Design review of the part built by this model. Coordinates are the model's own, in mm. A direction names the side the tool comes from. Give positions to 0.01 mm unless a question says otherwise; leave off trailing zeros. Write each loop counter-clockwise with the first axis right and the second up, starting at its lowest first coordinate (ties: lowest second). Pieces come first, ordered by that corner, then holes. Notation, with made-up numbers: M -38,66 L -29,66 A7 cw -29,78 Z; hole C -3,76.25 d3. An arc over 180 degrees is marked long. Answer in a Markdown table with one row per item.
```python
from build123d import *

# Parameters (mm, degrees)
F1_DEPTH = 63.5
F0_W     = 25.4
F0_H     = 19.05
F2_DEPTH = 25.4
F3_DEPTH = 7.9375
F5_R     = 6.35
F6_R     = 12.7
F7_DEPTH = 76.201
F8_R     = 2.54
F9_SIZE  = 2.54


with BuildPart() as f1:
    # F0 (on Front) → F1 (new body, symmetric)
    with BuildSketch(Plane.XZ):
        Polygon((-41.275, -9.525), (41.275, -9.525), (41.275, 9.525), (22.225, 9.525), (-41.275, 9.525), align=None)
    extrude(amount=F1_DEPTH, both=True)

    # F0 (on Front) → F2 (join, symmetric)
    with BuildSketch(Plane.XZ):
        with BuildLine():
            Line((22.225, 9.525), (41.275, 9.525))
            Line((41.275, 9.525), (41.275, 27.0002))
            ThreePointArc((41.275, 27.0002), (45.9246798487, 38.2255201513), (57.15, 42.8752))
            Line((57.15, 42.8752), (60.325, 42.8752))
            Line((60.325, 42.8752), (60.325, 61.9252))
            Line((60.325, 61.9252), (57.15, 61.9252))
            add(Edge.make_bspline(
                [(57.15, 61.9252), (56.6797844251, 61.9165132353), (56.2111060081, 61.9070782377), (55.7439674805, 61.896886054)],
                knots=[0, 0, 0, 0, 0.9174307887, 0.9174307887, 0.9174307887, 0.9174307887], degree=3))
            ThreePointArc((55.7439674805, 61.896886054), (31.9620930728, 51.1936902325), (22.225, 27.0002))
            Line((22.225, 27.0002), (22.225, 9.525))
        make_face()
        with Locations((73.025, 52.4002)):
            Rectangle(F0_W, F0_H)
    extrude(amount=F2_DEPTH, both=True)

    # F0 (on Front) → F3 (join, symmetric)
    with BuildSketch(Plane.XZ):
        with BuildLine():
            add(Edge.make_bspline(
                [(55.7439674805, 61.896886054), (-0.5649096696, 60.6683202624), (-34.4993601081, 48.437924622), (-41.275, 9.525)],
                knots=[0.9174307887, 0.9174307887, 0.9174307887, 0.9174307887, 111.5045361635, 111.5045361635, 111.5045361635, 111.5045361635], degree=3))
            Line((-41.275, 9.525), (22.225, 9.525))
            Line((22.225, 9.525), (22.225, 27.0002))
            ThreePointArc((22.225, 27.0002), (31.9620930728, 51.1936902325), (55.7439674805, 61.896886054))
        make_face()
    extrude(amount=F3_DEPTH, both=True)

    # F0 (on Front) → F4 (revolve)
    with BuildSketch(Plane.XZ):
        Polygon((85.725, 61.9252), (85.725, 42.8752), (85.725, 38.1), (111.125, 38.1), (111.125, 66.675), (85.725, 66.675), align=None)
    revolve(axis=Axis((85.725, 0, 52.3875), (0, 0, 1)))

    # F5
    f5_edges = [f1.edges().sort_by_distance(p)[0] for p in [
        (-41.275, -63.5, 0),
        (41.275, -63.5, 0),
        (41.275, 63.5, 0),
        (-41.275, 63.5, 0),
    ]]
    fillet(f5_edges, radius=F5_R)

    # F6 (on face) → F7 (cut, through all)
    with BuildSketch(Plane.XY.offset(66.675)):
        with Locations((85.725, 0)):
            Circle(F6_R)
    extrude(amount=-F7_DEPTH, mode=Mode.SUBTRACT)

    # F8
    f8_edges = [f1.edges().sort_by_distance(p)[0] for p in [
        (60.325, 0, 66.675),
        (60.325, 0, 38.1),
    ]]
    fillet(f8_edges, radius=F8_R)

    # F9
    f9_edges = [f1.edges().sort_by_distance(p)[0] for p in [
        (73.025, 0, 66.675),
        (73.025, 0, 38.1),
    ]]
    chamfer(f9_edges, length=F9_SIZE)


solid = f1.part
```
1) The part is to be moulded in two halves that separate along Y. For faces 1 (the face through (91.642, -11.376, 40.517)), 2 (the face through (46, 25.4, 42)), 3 (the face through (1, -36, 9.525)), say which applies: released by +Y, released by -Y, zero draft, split by the parting line, or undercut.
Geometry says:
| item | result |
|---|---|
| face 1 | undercut |
| face 2 | released by +Y |
| face 3 | zero draft |
2) For faces 4 (the face through (81, -15, 38.1)), 5 (the face through (46, -25.4, 42)), 6 (the face through (32.22, -16.79, 51.46)), 7 (the face through (45.8, -0.4, 38.1)), 8 (the face through (60, 2, 42.875)), list the 3-axis set-ups (+Z, -Z, +X, -X, +Y, -Y) from which the entire face can be reached by the end or side of a thin tool; tool diameter is ignored.
Geometry says:
| item | result |
|---|---|
| face 4 | -Z, +X, +Y, -Y |
| face 5 | +Z, +X, -X, -Y |
| face 6 | +Z, -X, -Y |
| face 7 | -Z, +Y, -Y |
| face 8 | -Z |
3) Insertion check: P1, Ø14.5, axis at x = 65, y = 8.5, coming from the -Z side; P2, Ø12, axis at x = 77.5, z = 50.5, coming from the +Y side; P3, Ø2, axis at x = -22, z = 27.5, coming from the -Y side. Each pin has a flat end and moves straight along its axis. Give the tip position at first contact, or say it passes through.
Geometry says:
| item | result |
|---|---|
| P1 | z = 38.1 |
| P2 | y = 25.4 |
| P3 | y = -7.94 |
4) Add section A-A (y = -36). Write out the cut boundary in (x, z) (3 decimals), and give its area (3 significant figures).
Geometry says:
| item | result |
|---|---|
| outline | M -41.275,-9.525 L 41.275,-9.525 L 41.275,9.525 L -41.275,9.525 Z |
| area | 1,570 mm^2 |
5) To check wall thickness, follow probe 1 along X at (y, z) = (21, 14.5) (3 decimals); probe 2 along Z at (x, y) = (35, -46.5) (3 decimals); probe 3 along Y at (x, z) = (25.5, 59.5). State the ranges of each line that lie inside material, in increasing order. Write a range as [from, to].
Geometry says:
| item | result |
|---|---|
| probe 1 | [22.225, 41.275] |
| probe 2 | [-9.525, 9.525] |
| probe 3 | [-7.94, 7.94] |
